Can you work these out from the model? Positions are in its coordinate system, mm. Face numbers are marked on the shaded views. A direction names the side the tool comes from. Round coordinates to 2 decimals unless told otherwise and drop trailing zeros. Write each loop counter-clockwise with the first axis right and the second up, starting at its lowest first coordinate (ties: lowest second). Pieces come first, ordered by that corner, then holes. Notation, with made-up numbers: (-6.5, 52) -> (36.5, 52) arc R9 ccw to (36.5, 62) -> close; hole circle Ø3 at (24.25, 13). An arc over 180 degrees is marked (long way). Write item = value, one per line. Start each with the question number.
1) If I drill on line 1 (Z direction, x = 34.5, y = 11.5); line 2 (Y direction, x = 35.5, z = 33.5), over which ranges is the centre line in solid material (lowest first)?
2) Thinking about a two-plate mould opening in Z: for the marked faces 1, 2, 3 and 4, which applies, +Z half, -Z half, draft (parallel to the pull), parting line (faces both ways), or undercut?
3) I'm going to push flat-ended pins straight in: pin 1 (1 mm diameter, centred on x = 18, y = 3.5, fed in from +Z); pin 2 (4 mm diameter, centred on y = 8.5, z = 45, fed in from -X); pin 3 (4 mm diameter, centred on x = 23, y = 16, fed in from -Z). Where does each tip first touch, or does it pass through?
4) Imagine slicing it at C-C, the plane x = 10. Please give me the cut outline in (y, z).
5) Imagine slicing it at D-D, the plane z = 21.5. Please give me the cut outline in (x, y), then the cut area to 3 significant figures.
6) Imagine slicing it at A-A, the plane z = 40. Please give me the cut outline in (x, y).
7) For the marked faces 5, 6 and 7, which set-ups out of +Z, -Z, +X, -X, +Y, -Y let a thin tool reach every point of the face, with its end or its side?
8) Imagine slicing it at B-B, the plane y = 13.5. Please give me the cut outline in (x, z), then the cut area to 3 significant figures.
from build123d import *

# Parameters (mm, degrees)
SKETCH1_W                = 20
SKETCH1_H                = 20
SKETCH1_W_2              = 16
SKETCH1_H_2              = 16
BOSS_EXTRUDE1_DEPTH      = 30
BOSS_EXTRUDE2_DEPTH      = 30
BOSS_EXTRUDE2_DEPTH_BACK = 20
SKETCH2_W                = 20
SKETCH2_H                = 20
SKETCH2_W_2              = 16
SKETCH2_H_2              = 16
SKETCH3_W                = 16
SKETCH3_H                = 16
CUT_EXTRUDE1_DEPTH       = 2
SKETCH4_W                = 16
SKETCH4_H                = 16
BOSS_EXTRUDE3_DEPTH      = 2
CHAMFER1_SIZE            = 1
BOSS_EXTRUDE4_REACH      = 83.243
SKETCH5_W                = 2
SKETCH5_H                = 20
BOSS_EXTRUDE6_REACH      = 83.243
SKETCH7_W                = 2
SKETCH7_H                = 20
FILLET1_R                = 10
FILLET2_R                = 3
CUT_EXTRUDE2_REACH       = 76.454
SKETCH8_R                = 2.25
FILLET3_R                = 5


with BuildPart() as part:
    # Sketch1 → Boss-Extrude1 (new body)
    with BuildSketch(Plane.XY):
        with Locations((10, 10)):
            Rectangle(SKETCH1_W, SKETCH1_H)
        with Locations((10, 10)):
            Rectangle(SKETCH1_W_2, SKETCH1_H_2, mode=Mode.SUBTRACT)
    extrude(amount=BOSS_EXTRUDE1_DEPTH)

    # Sketch2 → Boss-Extrude2 (add, two sides: drawn at the far end of the back side and taken through both)
    with BuildSketch(Plane(origin=(20, 0, 0), x_dir=(0, 0, -1), z_dir=(1, 0, 0)).offset(-BOSS_EXTRUDE2_DEPTH_BACK)):
        with Locations((-40, 10)):
            Rectangle(SKETCH2_W, SKETCH2_H)
        with Locations((-40, 10)):
            Rectangle(SKETCH2_W_2, SKETCH2_H_2, mode=Mode.SUBTRACT)
    extrude(amount=BOSS_EXTRUDE2_DEPTH + BOSS_EXTRUDE2_DEPTH_BACK)

    # Sketch3 → Cut-Extrude1 (cut)
    with BuildSketch(Plane(origin=(0, 0, 30), x_dir=(-1, 0, 0), z_dir=(0, 0, -1))):
        with Locations((-10, 10)):
            Rectangle(SKETCH3_W, SKETCH3_H)
    extrude(amount=-CUT_EXTRUDE1_DEPTH, mode=Mode.SUBTRACT)

    # Sketch4 → Boss-Extrude3 (add)
    with BuildSketch(Plane.ZY):
        with Locations((40, 10)):
            Rectangle(SKETCH4_W, SKETCH4_H)
    extrude(amount=-BOSS_EXTRUDE3_DEPTH)

    # Chamfer1
    chamfer1_edges = [part.edges().sort_by_distance(p)[0] for p in [
        (0, 10, 50),
    ]]
    chamfer(chamfer1_edges, length=CHAMFER1_SIZE)

    # Boss-Extrude4: up to this face of the body (flat: up to its plane)
    boss_extrude4_end = Plane(part.part.faces().sort_by_distance((0, 10, 24.5))[0])
    # Sketch5 → Boss-Extrude4 (add, up to the picked face)
    with BuildSketch(Plane(origin=(-24.5, 0, 24.5), x_dir=(0.7071067811865475, 0, 0.7071067811865477), z_dir=(-0.7071067811865477, 0, 0.7071067811865475)), mode=Mode.PRIVATE) as boss_extrude4_sk1:
        with Locations((33.648232278, 10)):
            Rectangle(SKETCH5_W, SKETCH5_H)
    boss_extrude4_tool1 = split(extrude(boss_extrude4_sk1.sketch, amount=-BOSS_EXTRUDE4_REACH, mode=Mode.PRIVATE), bisect_by=boss_extrude4_end, keep=Keep.BOTH, mode=Mode.PRIVATE)
    add(boss_extrude4_tool1.solids().sort_by(Axis((-0.707107, 10, 48.292893), (0.7071067811865477, 0, -0.7071067811865475)))[0])

    # Boss-Extrude6: up to this face of the body (flat: up to its plane)
    boss_extrude6_end = Plane(part.part.faces().sort_by_distance((25.5, 10, 50))[0])
    # Sketch7 → Boss-Extrude6 (add, up to the picked face)
    with BuildSketch(Plane(origin=(-24.5, 0, 24.5), x_dir=(0.7071067811865475, 0, 0.7071067811865477), z_dir=(-0.7071067811865477, 0, 0.7071067811865475)), mode=Mode.PRIVATE) as boss_extrude6_sk1:
        with Locations((37.062445841, 10)):
            Rectangle(SKETCH7_W, SKETCH7_H)
    boss_extrude6_tool1 = split(extrude(boss_extrude6_sk1.sketch, amount=-BOSS_EXTRUDE6_REACH, mode=Mode.PRIVATE), bisect_by=boss_extrude6_end, keep=Keep.BOTH, mode=Mode.PRIVATE)
    add(boss_extrude6_tool1.solids().sort_by(Axis((1.707107, 10, 50.707107), (0.7071067811865477, 0, -0.7071067811865475)))[0])

    # Fillet1
    # the kernel refuses this fillet: 10 mm, written as the material it adds along each edge
    with BuildSketch(Plane(origin=(0, 0, 46.171572875), x_dir=(-0.7071067811878772, 0, 0.7071067811852179), z_dir=(0, 1, 0))) as fillet1_piece_1:
        with BuildLine():
            CenterArc((4.445859456, -9.696276168), FILLET1_R, 104.157365729, 30.842634271)
            Line((-2.625208356, -2.625208356), (-2.766629712, -2.483787))
            Line((-2.766629712, -2.483787), (-0.141421356, 0.141421356))
            Line((-0.141421356, 0.141421356), (0, 0.2))
            ThreePointArc((0, 0.2), (1, 0.2), (1.951082811, 0.193925523))
            Line((1.951082811, 0.193925523), (2, 0))
        make_face()
    extrude(amount=20)
    with BuildSketch(Plane(origin=(3.828427125, 20, 50), x_dir=(1, 0, 0), z_dir=(0, -1, 0))) as fillet1_piece_2:
        with BuildLine():
            CenterArc((3.712605261, 10), FILLET1_R, 239.157365729, 30.842634271)
            Line((-1.414213562, 1.414213562), (-1.516749939, 1.242497834))
            ThreePointArc((-1.516749939, 1.242497834), (-0.848528137, 0.565685425), (-0.141421356, -0.141421356))
            Line((-0.141421356, -0.141421356), (0, -0.2))
            Line((0, -0.2), (3.712605261, -0.2))
            Line((3.712605261, -0.2), (3.712605261, 0))
        make_face()
    extrude(amount=20)

    # Fillet2
    fillet2_edges = [part.edges().sort_by_distance(p)[0] for p in [
        (18, 10, 32),
    ]]
    fillet(fillet2_edges, radius=FILLET2_R)

    # Cut-Extrude2: up to this face of the body (flat: up to its plane)
    cut_extrude2_end = Plane(part.part.faces().sort_by_distance((19.305922938, 0, 30.694077062))[0])
    # Sketch8 → Cut-Extrude2 (cut, up to the picked face)
    with BuildSketch(Plane(origin=(0, 20, 0), x_dir=(1, 0, 0), z_dir=(0, 1, 0)), mode=Mode.PRIVATE) as cut_extrude2_sk1:
        with Locations(Location((10, -40, 0), (0, 0, 270))):
            Circle(SKETCH8_R)
    cut_extrude2_tool1 = split(extrude(cut_extrude2_sk1.sketch, amount=-CUT_EXTRUDE2_REACH, mode=Mode.PRIVATE), bisect_by=cut_extrude2_end, keep=Keep.BOTH, mode=Mode.PRIVATE)
    add(cut_extrude2_tool1.solids().sort_by(Axis((10, 20, 40), (0, -1, 0)))[0], mode=Mode.SUBTRACT)

    # Fillet3
    fillet3_edges = [part.edges().sort_by_distance(p)[0] for p in [
        (20, 10, 30),
    ]]
    fillet(fillet3_edges, radius=FILLET3_R)


solid = part.part
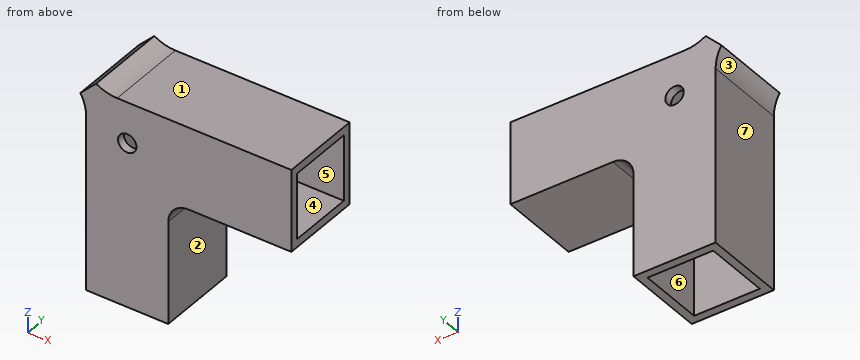
Reported:
q1.line_1 = 30 to 32, 48 to 50
q1.line_2 = 0 to 2, 18 to 20
q2.face_1 = +Z half
q2.face_2 = draft
q2.face_3 = -Z half
q2.face_4 = undercut
q3.pin_1 = 50
q3.pin_2 = -1.09
q3.pin_3 = 28
q4.outline = (0, 0) -> (2, 0) -> (2, 37.75) -> (0, 37.75) -> close; (0, 42.25) -> (2, 42.25) -> (2, 48) -> (18, 48) -> (18, 42.25) -> (20, 42.25) -> (20, 50) -> (0, 50) -> close; (18, 0) -> (20, 0) -> (20, 37.75) -> (18, 37.75) -> close
q5.outline = (0, 0) -> (20, 0) -> (20, 20) -> (0, 20) -> close; hole (2, 2) -> (18, 2) -> (18, 18) -> (2, 18) -> close
q5.area = 144 mm²
q6.outline = (0, 0) -> (7.75, 0) -> (7.75, 2) -> (2, 2) -> (2, 18) -> (7.75, 18) -> (7.75, 20) -> (0, 20) -> close; (12.25, 0) -> (50, 0) -> (50, 2) -> (12.25, 2) -> close; (12.25, 18) -> (50, 18) -> (50, 20) -> (12.25, 20) -> close
q7.face_5 = none
q7.face_6 = -Z
q7.face_7 = -Z, -X, +Y, -Y
q8.outline = (-1.41, 47.59) arc R10 cw to (0, 42.46) -> (0, 0) -> (2, 0) -> (2, 48) -> (50, 48) -> (50, 50) -> (7.54, 50) arc R10 cw to (2.41, 51.41) -> close; (18, 0) -> (20, 0) -> (20, 25) arc R5 cw to (25, 30) -> (50, 30) -> (50, 32) -> (21, 32) arc R3 ccw to (18, 29) -> close
q8.area = 330 mm²
